Geometry check sheet. Reference: the model listing, model coordinates, mm. Face numbers are marked on the shaded views. Round coordinates to 2 decimals unless told otherwise and drop trailing zeros. Order: outer loops, then holes, each group sorted by start corner. A loop starts at its lowest first (then second) coordinate and runs counter-clockwise, first axis right, second up. Notation, with made-up numbers: (-32, 81.25) -> (-22, 81.25) arc R23 ccw to (-22, 103.25) -> close; hole circle Ø6 at (80, 68.5). An arc over 180 degrees is marked (long way). Use a Markdown table: item, result. Add a question column.
Item 1: Mould release check, pull along Y, two halves, no side actions. Record for the marked faces 1 and 2: pulls with the +Y half, pulls with the -Y half, needs draft (parallel to the pull), parting line crosses it, or undercut.
Item 2: Material ranges on probe 1 along X at (y, z) = (-12, 1.35); probe 2 along Y at (x, z) = (80, 0.6); probe 3 along Y at (x, z) = (0, 0.75), recorded low to high. Write a range as [from, to].
Item 3: Sectioned sample at C-C, the plane x = 0. Record the cut outline in (y, z), and give its area (3 significant figures).
Item 4: Gauge pin test, flat ends, axial feed: pin 1 Ø6 at (x, y) = (32, 15) entering from -Z; pin 2 Ø1.5 at (y, z) = (59, -6) entering from -X; pin 3 Ø4 at (x, y) = (81, 69.5) entering from +Z. Record the tip position at first contact, or that the pin passes through.
Item 5: Sectioned sample at A-A, the plane x = 80. Record the cut outline in (y, z).
Item 6: Sectioned sample at B-B, the plane x = 24. Record the cut outline in (y, z).
Item 7: Sectioned sample at D-D, the plane y = 17. Record the cut outline in (x, z).
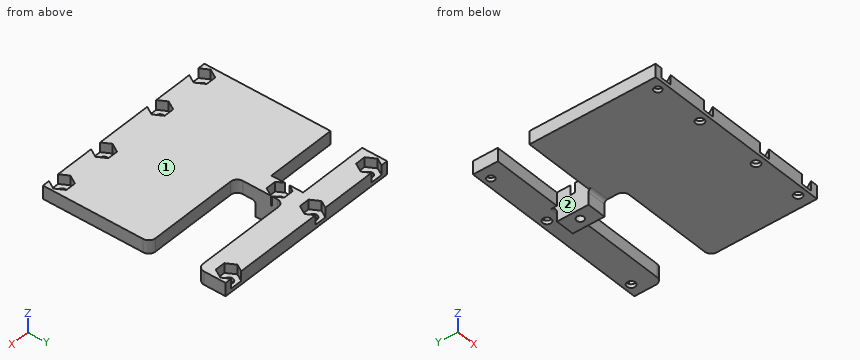
Autodesk Inventor part; units mm, degrees
ref_plane "Work Plane2" through (27.2145, 45.1271, -7.45) normal (0, 0, 1) x (1, 0, 0)
ref_plane "YZ Plane" through (0, 0, 0) normal (1, 0, 0) x (0, 1, 0)
ref_plane "XZ Plane" through (0, 0, 0) normal (0, 1, 0) x (-1, 0, 0)
ref_plane "Work Plane1" through (0, 0, 0) normal (0, 0, 1) x (1, 0, 0)
sketch "Sketch1" plane through (0, 0, 0) normal (0, 0, 1) x (1, 0, 0)
  line L0 (86, -8) -> (86, -12) construction
  line L1 (116, -16) -> (-164, -16) construction
  line L2 (116, 72) -> (-164, 72) construction
  line L3 (-6, 68) -> (-6, 64) construction
  line L4 (86, -16) -> (-6, -16)
  line L5 (-6, -16) -> (-6, 71.503)
  line L6 (-6, 71.503) -> (36.75, 71.503)
  line L7 (86, 35.181) -> (86, -16)
  line L8 (58.1676, 40.25) -> (85.5305, 40.25) construction
  line L9 (36.75, 47.9255) -> (36.75, 56.0811) construction
  line L10 (86, 35.181) -> (36.75, 35.181)
  line L11 (36.75, 35.181) -> (36.75, 58.041)
  line L12 (36.75, 71.503) -> (86, 71.503)
  line L13 (86, 71.503) -> (86, 58.041)
  line L14 (86, 58.041) -> (36.75, 58.041)
  point P0 (0, 0)
  dimension "d0" = 87.503
  dimension "d71" = 13.462
extrude "Extrusion1" add sketch "Sketch1" along normal blind 6.35
sketch "Sketch3" plane through (0, 0, 6.35) normal (0, 0, 1) x (1, 0, 0)
  circle A0 centre (32, 68) radius 2 construction
  point P0 (0, 0)
hole "Hole2" at (32, 68, 6.35) direction (0, 0, -1) diameter 3.9878 end through all
sketch "Sketch4" plane through (0, 0, 6.35) normal (0, 0, 1) x (1, 0, 0)
  circle A0 centre (80, -12) radius 2 construction
  circle A1 centre (80, -12) radius 4.8768 construction
  circle A2 centre (0, -12) radius 2 construction
  circle A3 centre (0, 68) radius 2 construction
  circle A4 centre (32, 68) radius 2 construction
  circle A5 centre (0, -12) radius 4.8768 construction
  circle A6 centre (0, 68) radius 1.9939 construction
  circle A7 centre (0, 68) radius 4.8768 construction
  circle A8 centre (32, 68) radius 1.9939 construction
  circle A9 centre (32, 68) radius 4.8768 construction
  circle A10 centre (24, -12) radius 2 construction
  circle A11 centre (56, -12) radius 2 construction
  circle A12 centre (56, -12) radius 4.8768 construction
  circle A13 centre (24, -12) radius 4.8768 construction
  circle A14 centre (80, -12) radius 1.9939
  line L0 (75.1232, -12) -> (77.5616, -7.7766)
  line L1 (77.5616, -7.7766) -> (82.4384, -7.7766)
  line L2 (82.4384, -7.7766) -> (84.8768, -12)
  line L3 (84.8768, -12) -> (82.4384, -16.2234)
  line L4 (82.4384, -16.2234) -> (77.5616, -16.2234)
  line L5 (77.5616, -16.2234) -> (75.1232, -12)
  line L6 (51.1232, -12) -> (53.5616, -7.7766)
  line L7 (53.5616, -7.7766) -> (58.4384, -7.7766)
  line L8 (58.4384, -7.7766) -> (60.8768, -12)
  line L9 (60.8768, -12) -> (58.4384, -16.2234)
  line L10 (58.4384, -16.2234) -> (53.5616, -16.2234)
  line L11 (53.5616, -16.2234) -> (51.1232, -12)
  line L12 (19.1232, -12) -> (21.5616, -7.7766)
  line L13 (21.5616, -7.7766) -> (26.4384, -7.7766)
  line L14 (26.4384, -7.7766) -> (28.8768, -12)
  line L15 (28.8768, -12) -> (26.4384, -16.2234)
  line L16 (26.4384, -16.2234) -> (21.5616, -16.2234)
  line L17 (21.5616, -16.2234) -> (19.1232, -12)
  line L18 (-4.8768, -12) -> (-2.4384, -7.7766)
  line L19 (-2.4384, -7.7766) -> (2.4384, -7.7766)
  line L20 (2.4384, -7.7766) -> (4.8768, -12)
  line L21 (4.8768, -12) -> (2.4384, -16.2234)
  line L22 (2.4384, -16.2234) -> (-2.4384, -16.2234)
  line L23 (-2.4384, -16.2234) -> (-4.8768, -12)
  line L24 (27.1232, 68) -> (29.5616, 72.2234)
  line L25 (29.5616, 72.2234) -> (34.4384, 72.2234)
  line L26 (34.4384, 72.2234) -> (36.8768, 68)
  line L27 (36.8768, 68) -> (34.4384, 63.7766)
  line L28 (34.4384, 63.7766) -> (29.5616, 63.7766)
  line L29 (29.5616, 63.7766) -> (27.1232, 68)
  line L30 (-4.8768, 68) -> (-2.4384, 72.2234)
  line L31 (-2.4384, 72.2234) -> (2.4384, 72.2234)
  line L32 (2.4384, 72.2234) -> (4.8768, 68)
  line L33 (4.8768, 68) -> (2.4384, 63.7766)
  line L34 (2.4384, 63.7766) -> (-2.4384, 63.7766)
  line L35 (-2.4384, 63.7766) -> (-4.8768, 68)
  point P0 (0, 0)
  dimension "d18" = 9.7536
  dimension "d21" = 9.7536
  dimension "d22" = 9.7536
  dimension "d23" = 9.7536
  dimension "d24" = 9.7536
  dimension "d25" = 9.7536
extrude "Extrusion2" cut sketch "Sketch4" against normal blind 4.6228
sketch "Sketch5" plane through (0, 0, 6.35) normal (0, 0, 1) x (1, 0, 0)
  circle A0 centre (56, -12) radius 2 construction
  circle A1 centre (24, -12) radius 2 construction
  point P0 (0, 0)
hole "Hole3" at (56, -12, 6.35) at (24, -12, 6.35) direction (0, 0, -1) diameter 3.9878 end through all
sketch "Sketch6" plane through (0, 0, 6.35) normal (0, 0, 1) x (1, 0, 0)
  circle A0 centre (32, 52) radius 1.8 construction
  line L0 (25.6709, 58.1897) -> (15.8763, 58.1897) construction
  line L1 (15.8763, 45.8103) -> (25.6716, 45.8103) construction
  line L2 (26.268, 46.528) -> (26.268, 49.5214) construction
  line L3 (5.9638, 51.1237) -> (5.9638, 48.0771) construction
  circle A1 centre (32, 52) radius 1.778
  circle A2 centre (32, 52) radius 4.8768 construction
  line L4 (27.1232, 52) -> (29.5616, 56.2234)
  line L5 (29.5616, 56.2234) -> (34.4384, 56.2234)
  line L6 (34.4384, 56.2234) -> (36.8768, 52)
  line L7 (36.8768, 52) -> (34.4384, 47.7766)
  line L8 (34.4384, 47.7766) -> (29.5616, 47.7766)
  line L9 (29.5616, 47.7766) -> (27.1232, 52)
  line L10 (26.268, 45.875) -> (5.9638, 45.875)
  line L11 (5.9638, 45.875) -> (5.9638, 58.1897)
  line L12 (5.9638, 58.1897) -> (26.268, 58.1897)
  line L13 (26.268, 58.1897) -> (26.268, 45.875)
  line L14 (4.5388, 44.45) -> (27.693, 44.45)
  line L15 (27.693, 44.45) -> (27.693, 59.6147)
  line L16 (27.693, 59.6147) -> (4.5388, 59.6147)
  line L17 (4.5388, 59.6147) -> (4.5388, 44.45)
  line L18 (27.693, 44.45) -> (4.5388, 44.45)
  line L19 (4.5388, 44.45) -> (4.5388, 59.6147)
  line L20 (4.5388, 59.6147) -> (27.693, 59.6147)
  line L21 (27.693, 59.6147) -> (27.693, 44.45)
  line L22 (-6, 71.503) -> (-6, -16) construction
  line L23 (4.5388, 59.6147) -> (-6, 59.6147)
  line L24 (-6, 59.6147) -> (-6, 44.45)
  line L25 (-6, 44.45) -> (4.5388, 44.45)
  line L26 (4.5388, 44.45) -> (4.5388, 59.6147)
  circle A3 centre (0, -12) radius 2 construction
  circle A4 centre (0, 68) radius 2 construction
  circle A5 centre (80, -12) radius 2 construction
  point P0 (0, 0)
  dimension "d36" = 9.7536
  dimension "d35" = 3.556
  dimension "d48" = 1.425
hole "Hole4" at (32, 52, 6.35) direction (0, 0, -1) diameter 3.556 end through all
extrude "Extrusion3" cut sketch "Sketch6" against normal blind 4.6228 contours L4 L15 L9 | L4 L5 L6 L7 L8 L9 L15
extrude "Extrusion4" cut sketch "Sketch6" against normal through all contours L10 L11 L12 L13
extrude "Extrusion5" cut sketch "Sketch6" against normal through all contours L9 L15 L14 L17 L16 L4 | L4 L15 L9
sketch "Sketch7" plane through (0, 0, 0) normal (0, 0, -1) x (-1, 0, 0)
  line L0 (-27.693, 59.6147) -> (-4.5388, 59.6147)
  line L1 (-4.5388, 59.6147) -> (-4.5388, 44.45)
  line L2 (-4.5388, 44.45) -> (-27.693, 44.45)
  line L3 (-27.693, 44.45) -> (-27.693, 59.6147)
  circle A0 centre (-32, 52) radius 1.778
  circle A1 centre (-56, -12) radius 1.9939
  circle A2 centre (-24, -12) radius 1.9939
  circle A3 centre (-32, 68) radius 1.9939
  line L4 (-86, -16) -> (6, -16)
  line L5 (6, -16) -> (6, 71.503)
  line L6 (6, 71.503) -> (-86, 71.503)
  line L7 (-36.75, 58.041) -> (-36.75, 35.181)
  line L8 (-36.75, 35.181) -> (-86, 35.181)
  line L9 (-86, 35.181) -> (-86, -16)
  line L10 (1.3245, 44.5) -> (-33.3311, 44.5) construction
  line L11 (-33.3245, 59.5) -> (1.3311, 59.5) construction
  line L12 (-27.693, 44.45) -> (-27.693, 59.6147) construction
  line L13 (-27.693, 44.45) -> (-4.5388, 44.45)
  line L14 (-36.75, 52.2196) -> (-36.75, 58.041)
  line L15 (-27.693, 44.45) -> (-36.75, 44.45)
  line L16 (-36.75, 44.45) -> (-36.75, 59.6147)
  line L17 (-36.75, 59.6147) -> (-27.693, 59.6147)
  line L18 (-27.693, 59.6147) -> (-27.693, 44.45)
  line L19 (-86, 71.503) -> (-86, 58.041)
  line L20 (-86, 58.041) -> (-36.75, 58.041)
  point P0 (0, 0)
  point P1 (-36.75, 67.7804)
ref_plane "Work Plane2" through (27.2145, 45.1271, -7.45) normal (0, 0, 1) x (1, 0, 0)
extrude "Extrusion6" add sketch "Sketch7" along normal up to surface (7.45 mm away) contours L3 L15 L7 L16 L17
sketch "Sketch8" plane through (-6, -16, 0) normal (-1, 0, 0) x (0, 0, 1)
  point P0 (0, 16)
extrude "Extrusion7" cut sketch "Sketch6" against normal through all contours L17 L25 L24 L23
hole "Hole5" at (80, -12, 6.35) at (0, -12, 6.35) at (0, 68, 6.35) direction (0, 0, -1) diameter 3.556 end through all
fillet "Fillet1" radius 1.524 1 edges at (32.2215, 44.45, 0)
fillet "Fillet2" radius 3.175 3 edges at (32.2215, 59.6147, 0) (36.75, 35.181, 3.175) (86, 35.181, 3.175)
hole "Hole6" at (80, -12, 6.35) direction (0, 0, -1) diameter 3.9878 end through all
fillet "Fillet3" radius 3.175 1 edges at (86, 58.041, 3.175)
fillet "Fillet4" radius 3.175 1 edges at (36.75, 58.041, 3.175)
sketch "Sketch9" plane through (0, 0, 6.35) normal (0, 0, 1) x (1, 0, 0)
  circle A0 centre (80, 68) radius 2 construction
  circle A1 centre (80, 68) radius 4.8768 construction
  line L0 (75.1232, 68) -> (77.5616, 72.2234)
  line L1 (77.5616, 72.2234) -> (82.4384, 72.2234)
  line L2 (82.4384, 72.2234) -> (84.8768, 68)
  line L3 (84.8768, 68) -> (82.4384, 63.7766)
  line L4 (82.4384, 63.7766) -> (77.5616, 63.7766)
  line L5 (77.5616, 63.7766) -> (75.1232, 68)
  circle A2 centre (80, 68) radius 1.9939
  point P0 (0, 0)
  dimension "d74" = 9.7536
  dimension "d75" = 3.9878
extrude "Extrusion8" cut sketch "Sketch9" against normal through all contours A2
sketch "Sketch10" plane through (0, 0, 6.35) normal (0, 0, 1) x (1, 0, 0)
  circle A0 centre (80, 68) radius 1.9939 construction
  circle A1 centre (80, 68) radius 4.8768 construction
  line L0 (75.1232, 68) -> (77.5616, 72.2234)
  line L1 (77.5616, 72.2234) -> (82.4384, 72.2234)
  line L2 (82.4384, 72.2234) -> (84.8768, 68)
  line L3 (84.8768, 68) -> (82.4384, 63.7766)
  line L4 (82.4384, 63.7766) -> (77.5616, 63.7766)
  line L5 (77.5616, 63.7766) -> (75.1232, 68)
  point P0 (0, 0)
  dimension "d78" = 9.7536
extrude "Extrusion9" cut sketch "Sketch10" against normal blind 4.6228
properties part number "SensorWall"
Found:
| question | item | result |
|---|---|---|
| 1 | face 1 | needs draft |
| 1 | face 2 | undercut |
| 2 | probe 1 | x = [-6, -1.78], [1.78, 22.01], [25.99, 54.01], [57.99, 78.01], [81.99, 86] |
| 2 | probe 2 | y = [-16, -13.99], [-10.01, 35.18], [58.04, 66.01], [69.99, 71.5] |
| 2 | probe 3 | y = [-16, -13.78], [-10.22, 44.45], [59.61, 66.22], [69.78, 71.5] |
| 3 | outline | (-16, 0) -> (-13.78, 0) -> (-13.78, 1.73) -> (-16, 1.73) -> close; (-10.22, 0) -> (44.45, 0) -> (44.45, 6.35) -> (-7.78, 6.35) -> (-7.78, 1.73) -> (-10.22, 1.73) -> close; (59.61, 0) -> (66.22, 0) -> (66.22, 1.73) -> (63.78, 1.73) -> (63.78, 6.35) -> (59.61, 6.35) -> close; (69.78, 0) -> (71.5, 0) -> (71.5, 1.73) -> (69.78, 1.73) -> close |
| 3 | area | 373 mm2 |
| 4 | pin 1 | stops at z = 0 |
| 4 | pin 2 | stops at x = 27.69 |
| 4 | pin 3 | stops at z = 1.73 |
| 5 | outline | (-16, 0) -> (-13.99, 0) -> (-13.99, 1.73) -> (-16, 1.73) -> close; (-10.01, 0) -> (35.18, 0) -> (35.18, 6.35) -> (-7.78, 6.35) -> (-7.78, 1.73) -> (-10.01, 1.73) -> close; (58.04, 0) -> (66.01, 0) -> (66.01, 1.73) -> (63.78, 1.73) -> (63.78, 6.35) -> (58.04, 6.35) -> close; (69.99, 0) -> (71.5, 0) -> (71.5, 1.73) -> (69.99, 1.73) -> close |
| 6 | outline | (-16, 0) -> (-13.99, 0) -> (-13.99, 1.73) -> (-16, 1.73) -> close; (-10.01, 0) -> (44.45, 0) -> (44.45, 6.35) -> (-7.78, 6.35) -> (-7.78, 1.73) -> (-10.01, 1.73) -> close; (59.61, 0) -> (71.5, 0) -> (71.5, 6.35) -> (59.61, 6.35) -> close |
| 7 | outline | (-6, 0) -> (86, 0) -> (86, 6.35) -> (-6, 6.35) -> close |
